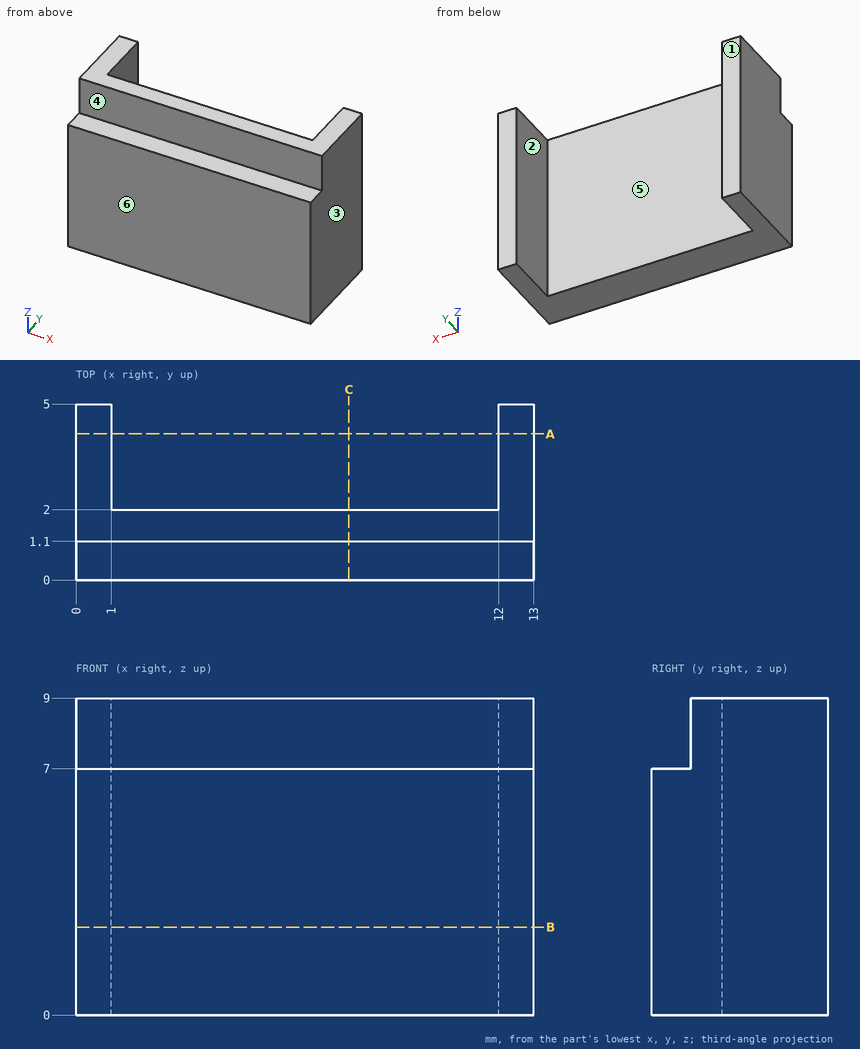
Geometry: see drawing. Coordinates: mm, zero at the bounding-box minimum. A direction names the side the tool comes from. Give positions to 0.01 mm unless a question says otherwise; leave off trailing zeros. Write each loop counter-clockwise with the first axis right and the second up, starting at its lowest first coordinate (ties: lowest second). Pieces come first, ordered by that corner, then holes. Notation, with made-up numbers: M -31.75,-33 L 4.25,-33 A8 cw 4.25,-25 Z; hole C 13,0 d11. An arc over 180 degrees is marked long. Return JSON: item names as keys, results as strings. Group by question number.
1) Cut plane A-A, the plane y = 4.15. Output: boundary loops of the cut face in (x, z).
2) First-contact query: pin 1 Ø0.6 at (x, y) = (9, 0.5) entering from +Z; pin 2 Ø4.5 at (x, z) = (8.5, 6.5) entering from +Y; pin 3 Ø1.6 at (x, z) = (6.5, 8) entering from -Y. Flat tips, straight axial feed; report the tip coordinate or a pass-through.
3) Cut plane B-B, the plane z = 2.5. Output: boundary loops of the cut face in (x, y).
4) Draft query along X for the marked faces 1, 2 and 3. Return one class per face: released by +X, released by -X, zero draft, split by the parting line, or undercut.
5) Set-up query: the marked faces 4, 5 and 6. Return all of +Z, -Z, +X, -X, +Y, -Y with unobstructed straight access to the full face (end or side cutting, diameter ignored); none if empty.
6) Cut plane C-C, the plane x = 7.75. Output: boundary loops of the cut face in (y, z).
7) Ray query, L1, parallel to X at y = 2.8, z = 7; L2, parallel to Y at x = 9.5, z = 3.75; L3, parallel to Z at x = 4.75, y = 0.5. Return the intervals inside material, ascending.
Data:
{
 "1": {"outline": "M 0,0 L 1,0 L 1,9 L 0,9 Z; M 12,0 L 13,0 L 13,9 L 12,9 Z"},
 "2": {"pin 1": "stops at z = 7", "pin 2": "stops at y = 2", "pin 3": "stops at y = 1.1"},
 "3": {"outline": "M 0,0 L 13,0 L 13,5 L 12,5 L 12,2 L 1,2 L 1,5 L 0,5 Z"},
 "4": {"face 1": "zero draft", "face 2": "undercut", "face 3": "released by +X"},
 "5": {"face 4": "+Z, +X, -X, -Y", "face 5": "+Z, -Z, +Y", "face 6": "+Z, -Z, +X, -X, -Y"},
 "6": {"outline": "M 0,0 L 2,0 L 2,9 L 1.1,9 L 1.1,7 L 0,7 Z"},
 "7": {"L1": "x = 0 to 1, 12 to 13", "L2": "y = 0 to 2", "L3": "z = 0 to 7"}
}
